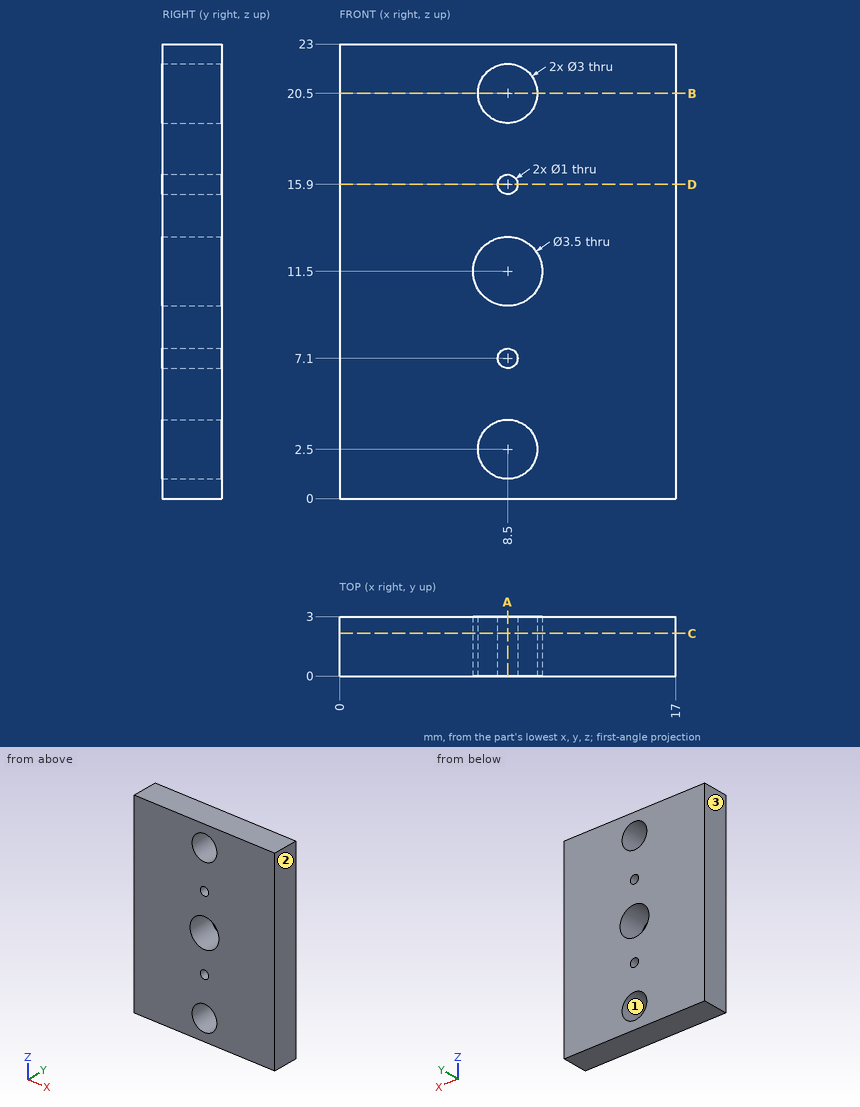
Job drawing, mm, ordinate dimensions from the low corner. One solid piece. Give positions to 0.01 mm unless a question says otherwise; leave off trailing zeros. Write each loop counter-clockwise with the first axis right and the second up, starting at its lowest first coordinate (ties: lowest second). Pieces come first, ordered by that corner, then holes. Notation, with made-up numbers: M -15.75,82 L 13.25,82 A31 cw 13.25,109 Z; hole C 16,73.25 d6. An arc over 180 degrees is marked long. One line per item, written item: value. Start each with the question number.
Q1. Saw through at A-A, the plane x = 8.5. Write the cut outline in (y, z).
Q2. Saw through at B-B, the plane z = 20.5. Write the cut outline in (x, y), plus the area to 3 significant figures.
Q3. Probe probe 1 along Z at (x, y) = (8.5, 1.25); probe 2 along X at (y, z) = (1.2, 11.5); probe 3 along X at (y, z) = (1.7, 15.9). List the from-to ranges inside material, lowest first. Write a range as [from, to].
Q4. Saw through at D-D, the plane z = 15.9. Write the cut outline in (x, y).
Q5. Drop a flat-ended pin along its axis: pin 1 Ø2.5 at (x, z) = (8.5, 2.5) entering from +Y. Give the stop position or say it passes through.
Q6. Saw through at C-C, the plane y = 2.15. Write the cut outline in (x, z), plus the area to 3 significant figures.
Q7. Two-plate mould, pull along X, no slides. Class the marked faces 1, 2 and 3: +X half, -X half, draft (parallel to the pull), parting line (faces both ways), or undercut.
Output values:
1. outline: M 0,0 L 3,0 L 3,1 L 0,1 Z; M 0,4 L 3,4 L 3,6.6 L 0,6.6 Z; M 0,7.6 L 3,7.6 L 3,9.75 L 0,9.75 Z; M 0,13.25 L 3,13.25 L 3,15.4 L 0,15.4 Z; M 0,16.4 L 3,16.4 L 3,19 L 0,19 Z; M 0,22 L 3,22 L 3,23 L 0,23 Z
2. outline: M 0,0 L 7,0 L 7,3 L 0,3 Z; M 10,0 L 17,0 L 17,3 L 10,3 Z
2. area: 42.0 mm²
3. probe 1: z = [0, 1], [4, 6.6], [7.6, 9.75], [13.25, 15.4], [16.4, 19], [22, 23]
3. probe 2: x = [0, 6.75], [10.25, 17]
3. probe 3: x = [0, 8], [9, 17]
4. outline: M 0,0 L 8,0 L 8,3 L 0,3 Z; M 9,0 L 17,0 L 17,3 L 9,3 Z
5. pin 1: passes through
6. outline: M 0,0 L 17,0 L 17,23 L 0,23 Z; hole C 8.5,11.5 d3.5; hole C 8.5,2.5 d3; hole C 8.5,20.5 d3; hole C 8.5,7.1 d1; hole C 8.5,15.9 d1
6. area: 366 mm²
7. face 1: undercut
7. face 2: +X half
7. face 3: -X half
